Autodesk Inventor part; units mm, degrees
ref_plane "YZ Plane" through (0, 0, 0) normal (1, 0, 0) x (0, 1, 0)
ref_plane "XZ Plane" through (0, 0, 0) normal (0, 1, 0) x (-1, 0, 0)
ref_plane "XY Plane" through (0, 0, 0) normal (0, 0, 1) x (1, 0, 0)
sketch "Sketch1" plane through (0, 0, 0) normal (0, 0, 1) x (1, 0, 0)
  line L0 (-2.5, -0.5) -> (2.5, -0.5)
  line L1 (2.5, -0.5) -> (2.5, 2.5)
  line L2 (2.5, 2.5) -> (-2.5, 2.5)
  line L3 (-2.5, 2.5) -> (-2.5, -0.5)
  line L4 (-2.5, -0.5) -> (2.5, 2.5) construction
  line L5 (2.5, -0.5) -> (-2.5, 2.5) construction
  point P0 (0, 0)
  point P1 (0, 1)
  dimension "d0" = 5
  dimension "d1" = 3
  dimension "d10" = 1
  dimension "d11" = 0
extrude "Extrusion1" add sketch "Sketch1" along normal mid plane 3.8
sketch "Sketch2" plane through (0, 0, 0) normal (0, 0, 1) x (1, 0, 0)
  line L0 (0, 0) -> (-2, 0)
  line L1 (-2, 0) -> (-2, -1.46)
  line L2 (-2, -1.46) -> (-2.54, -2)
  line L3 (-2.54, -2) -> (-2.54, -5)
  line L4 (0, 0) -> (0, -4.5028) construction
  line L5 (0, 0) -> (2, 0)
  line L6 (2, 0) -> (2, -1.46)
  line L7 (2, -1.46) -> (2.54, -2)
  line L8 (2.54, -2) -> (2.54, -5)
  dimension "d4" = 3
  dimension "d5" = 2.54
  dimension "d6" = 45
  dimension "d8" = 2
  dimension "d9" = 2
fillet "Fillet1" radius 1 12 edges at (0, -0.5, -1.9) (-2.5, 1, -1.9) (0, 2.5, -1.9) (2.5, 1, -1.9) (-2.5, -0.5, 0) (-2.5, 1, 1.9) (-2.5, 2.5, 0) (0, 2.5, 1.9) (2.5, 2.5, 0) (2.5, 1, 1.9) (2.5, -0.5, 0) (0, -0.5, 1.9)
sketch "Sketch3" plane through (0, 0, 0) normal (1, 0, 0) x (0, 1, 0)
  circle A0 centre (0, 0) radius 0.25
  dimension "d13" = 0.5
sweep "Sweep1" add profiles "Sketch3" path "Sketch2"
properties part number "Capacitor"
Can you work these out from the model? Positions are in its coordinate system, mm. A direction names the side the tool comes from. Give positions to 0.01 mm unless a question says otherwise; leave off trailing zeros. Write each loop counter-clockwise with the first axis right and the second up, starting at its lowest first coordinate (ties: lowest second). Pieces come first, ordered by that corner, then holes. Notation, with made-up numbers: (58, 84.5) -> (110, 84.5) arc R24 ccw to (110, 111.5) -> close; hole circle Ø1 at (84, 42). An arc over 180 degrees is marked (long way). Answer as a JSON object with one key per item and string values. Group by question number.
Item 1: Suppose I cut it at A-A (z = -1.5). Please give me the cut outline in (x, y).
Item 2: For faces 1 (the face through (0, -0.5, 0)), 2 (the face through (2.5, 1, 0)), 3 (the face through (-0.021, 2.199, 1.615)), 4 (the face through (-2.5, 1, 0)), 5 (the face through (-2.199, 0.993, 1.615)), which set-ups out of +Z, -Z, +X, -X, +Y, -Y let a thin tool reach every point of the face, with its end or its side?
Item 3: Suppose I cut it at B-B (y = -3.5). Please give me the cut outline in (x, z).
Item 4: Suppose I cut it at C-C (x = 0). Please give me the cut outline in (y, z), plus the area to 3 significant figures.
Item 5: We'd pull the mould along Y, two halves only. Please class faces 6 (the face through (2.215, 1.007, -1.599)), 7 (the face through (-2.33, -0.06, 0.21)), 8 (the face through (-2.215, 2.199, -0.013)): +Y half, -Y half, draft (parallel to the pull), parting line (faces both ways), or undercut.
Item 6: I'm going to push flat-ended pins straight in: P1, Ø0.5, axis at y = 1, z = 0, coming from the +X side; P2, Ø0.5, axis at y = 1, z = -0.5, coming from the -X side; P3, Ø0.9, axis at x = 0.5, z = 0.5, coming from the -Y side. Where does each tip first touch, or does it pass through?
Item 7: Please list where these lines run through material, in increasing order: line 1 (Y direction, x = 1.2, z = 0); line 2 (X direction, y = 1.5, z = -0.5); line 3 (Z direction, x = -1.55, y = 0.5). Write a range as [from, to].
Findings:
{
 "1": {"outline": "(-2.3, 0.5) arc R0.8 ccw to (-1.5, -0.3) -> (1.5, -0.3) arc R0.8 ccw to (2.3, 0.5) -> (2.3, 1.5) arc R0.8 ccw to (1.5, 2.3) -> (-1.5, 2.3) arc R0.8 ccw to (-2.3, 1.5) -> close"},
 "2": {"face 1": "+Z, -Z, -Y", "face 2": "+Z, -Z, +X, +Y", "face 3": "+Z, +X, -X, +Y", "face 4": "+Z, -Z, -X, +Y", "face 5": "+Z, -X, +Y, -Y"},
 "3": {"outline": "circle Ø0.5 at (-2.54, 0); circle Ø0.5 at (2.54, 0)"},
 "4": {"outline": "(-0.5, -0.9) arc R1 ccw to (0.5, -1.9) -> (1.5, -1.9) arc R1 ccw to (2.5, -0.9) -> (2.5, 0.9) arc R1 ccw to (1.5, 1.9) -> (0.5, 1.9) arc R1 ccw to (-0.5, 0.9) -> close", "area": "10.5 mm²"},
 "5": {"face 6": "draft", "face 7": "undercut", "face 8": "+Y half"},
 "6": {"P1": "stops at x = 2.5", "P2": "stops at x = -2.5", "P3": "stops at y = -0.5"},
 "7": {"line 1": "y = [-0.5, 2.5]", "line 2": "x = [-2.5, 2.5]", "line 3": "z = [-1.9, 1.9]"}
}
